CAD build for the part. Positions are in the model's coordinates, mm. A direction names the side the tool comes from. Coordinates: 2 decimals unless noted, no trailing zeros. Write each loop counter-clockwise with the first axis right and the second up, starting at its lowest first coordinate (ties: lowest second). Pieces come first, ordered by that corner, then holes.
```python
from build123d import *
from OCP.BRepFilletAPI import BRepFilletAPI_MakeFillet

# Parameters (mm, degrees)
SKETCH1_W           = 8.4
SKETCH1_H           = 23.5
BOSS_EXTRUDE1_DEPTH = 1
SKETCH1_3_W         = 11.6
SKETCH1_3_H         = 23.5
BOSS_EXTRUDE4_DEPTH = 1
BOSS_EXTRUDE5_START = -1
BOSS_EXTRUDE5_DEPTH = 9.4
FILLET2_R           = 1
FILLET2_R_2         = 0.8
FILLET3_R           = 5
CUT_EXTRUDE1_START  = -6
SKETCH4_R           = 0.902238409
CUT_EXTRUDE1_DEPTH  = 7
BOSS_EXTRUDE8_DEPTH = 1


# Read off the part's stored shape, not the designer's step: Mirror1
with BuildPart() as part:
    # Sketch1 → Boss-Extrude1 (new body)
    with BuildSketch(Plane.XY):
        Rectangle(SKETCH1_W, SKETCH1_H)
    extrude(amount=BOSS_EXTRUDE1_DEPTH)

    # Sketch1<3> → Boss-Extrude4 (add)
    with BuildSketch(Plane.XY):
        with Locations((-10, 0)):
            Rectangle(SKETCH1_3_W, SKETCH1_3_H)
    extrude(amount=BOSS_EXTRUDE4_DEPTH)

    # Sketch3 → Boss-Extrude5 (add)
    with BuildSketch(Plane(origin=(0, 0, 0), x_dir=(-1, 0, 0), z_dir=(0, 0, -1)).offset(BOSS_EXTRUDE5_START)):
        Polygon((0.05, 8.9), (7.05, 8.9), (7.05, 11.75), (5.05, 11.75), (5.05, 9.9), (0.05, 9.9), align=None)
        Polygon((7.8, 11.75), (7.8, 8.9), (14.8, 8.9), (14.8, 9.9), (9.8, 9.9), (9.8, 11.75), align=None)
    extrude(amount=BOSS_EXTRUDE5_DEPTH)

    # Fillet2
    fillet2_edges_1 = [part.edges().sort_by_distance(p)[0] for p in [
        (-9.8, 11.75, -4.2),
        (-5.05, 11.75, -4.2),
        (-0.05, 9.9, -4.2),
        (-14.8, 9.9, -4.2),
    ]]
    fillet2_edges_2 = [part.edges().sort_by_distance(p)[0] for p in [
        (-9.8, 9.9, -4.2),
        (-5.05, 9.9, -4.2),
    ]]
    fillet2 = BRepFilletAPI_MakeFillet(part.part.solid().wrapped)
    for e in fillet2_edges_1:
        fillet2.Add(FILLET2_R - 0.0001, e.wrapped)
    for e in fillet2_edges_2:
        fillet2.Add(FILLET2_R_2 - 0.0001, e.wrapped)
    add(Compound.cast(fillet2.Shape()), mode=Mode.REPLACE)  # a hair under: the kernel refuses the full size

    # Fillet3
    fillet3_edges = [part.edges().sort_by_distance(p)[0] for p in [
        (-15.8, 11.75, 0.5),
        (-15.8, -11.75, 0.5),
        (4.2, -11.75, 0.5),
        (4.2, 11.75, 0.5),
    ]]
    fillet(fillet3_edges, radius=FILLET3_R)

    # Sketch4 → Cut-Extrude1 (cut)
    with BuildSketch(Plane.ZY.offset(9.8).offset(CUT_EXTRUDE1_START)):
        with Locations(Location((-4.2, 10.05, 0), (0, 0, 189.57004168))):
            Circle(SKETCH4_R)
    extrude(amount=CUT_EXTRUDE1_DEPTH, mode=Mode.SUBTRACT)

    # Mirror1: part across plane


with BuildPart() as part_1:
    add(part.part)
    add(part.part.mirror(Plane.ZX))

    # Sketch7 → Boss-Extrude8 (add)
    with BuildSketch(Plane.XY):
        with BuildLine():
            Line((-1.8, 15), (-19.8, 15))
            ThreePointArc((-19.8, 15), (-24.042640687, 13.242640687), (-25.8, 9))
            Line((-25.8, 9), (-25.8, -9))
            ThreePointArc((-25.8, -9), (-24.042640687, -13.242640687), (-19.8, -15))
            Line((-19.8, -15), (-1.8, -15))
            ThreePointArc((-1.8, -15), (2.442640687, -13.242640687), (4.2, -9))
            Line((4.2, -9), (4.2, 9))
            ThreePointArc((4.2, 9), (2.442640687, 13.242640687), (-1.8, 15))
        make_face()
    extrude(amount=BOSS_EXTRUDE8_DEPTH)


solid = part_1.part
```
Item 1: Which spindle directions (+Z, -Z, +X, -X, +Y, -Y) get a long thin tool onto all of the face, cutting with end or side? Do faces 4 (the cylindrical face through (-5.351, -11.465, -4.259)), 5 (the cylindrical face through (-9.499, 11.465, -4.259)), 6 (the cylindrical face through (-9.499, -11.465, -4.259)). Say none if no direction does.
Item 2: Saw through at C-C, the plane y = -3.75. Write the cut outline in (x, z), and give its area (3 significant figures).
Item 3: Wall check: line 1 along Z through (x, y) = (-8.4, -10.05); line 2 along Y through (x, z) = (-9.9, -4.2); line 3 along Y through (x, z) = (-13, -3.75). Give the ranges that are in metal, low to high.
Item 4: Saw through at A-A, the plane x = -3.25. Write the cut outline in (y, z).
Item 5: Saw through at D-D, the plane x = -17. Write the cut outline in (y, z), and give its area (3 significant figures).
Item 6: Saw through at B-B, the plane z = -2.75. State how many separate pieces and enclosed holes the cut face has, and give its area (3 significant figures).
Item 7: Two-plate mould, pull along X, no slides. Class faces 1 (the cylindrical face through (-14.499, -9.615, -4.259)), 2 (the flat face through (-8, 11.75, -4)), 3 (the flat face through (-7.8, -10, -3)): +X half, -X half, draft (parallel to the pull), parting line (faces both ways), or undercut.
Item 8: Flat gauge pins, fed straight in: pin 1 Ø5.5 at (x, z) = (-10, -4.5) entering from +Y; pin 2 Ø1.6 at (x, z) = (-3.5, -2.5) entering from +Y; pin 3 Ø1.6 at (y, z) = (-10.05, -4.2) entering from -X; pin 4 Ø5 at (y, z) = (-4.5, -0.5) entering from +X. Where does each tip first touch, or does it go through?
Working result:
1. face 4: -Z, +X, -Y
1. face 5: -Z, -X, +Y
1. face 6: -Z, -X, -Y
2. outline: (-25.8, 0) - (4.2, 0) - (4.2, 1) - (-25.8, 1) - close
2. area: 30.0 mm2
3. line 1: z = -8.4 to -5.1, -3.3 to 1
3. line 2: y = -9.15 to -8.9, 8.9 to 9.15
3. line 3: y = -9.9 to -8.9, 8.9 to 9.9
4. outline: (-15, 0) - (-9.9, 0) - (-9.9, -8.4) - (-8.9, -8.4) - (-8.9, 0) - (8.9, 0) - (8.9, -8.4) - (9.9, -8.4) - (9.9, 0) - (15, 0) - (15, 1) - (-15, 1) - close
5. outline: (-15, 0) - (15, 0) - (15, 1) - (-15, 1) - close
5. area: 30.0 mm2
6. separate pieces: 4
6. enclosed holes: 0
6. area: 41.6 mm2
7. face 1: -X half
7. face 2: draft
7. face 3: undercut
8. pin 1: stops at y = 11.75
8. pin 2: stops at y = 9.9
8. pin 3: stops at x = -14.74
8. pin 4: stops at x = 4.2
